Source: CAD feature listing. Evaluate the final solid. Frame: model axes, mm. Face numbers are marked on the shaded views. Coordinates: 2 decimals unless noted, no trailing zeros. Write each loop counter-clockwise with the first axis right and the second up, starting at its lowest first coordinate (ties: lowest second). Pieces come first, ordered by that corner, then holes. Notation, with made-up numbers: (66.25, 65) - (72.25, 65) arc R19 cw to (72.25, 101) - close; hole circle Ø7 at (-27, -2). An arc over 180 degrees is marked (long way). One line per question, with ' | ' between items. Start each with the question number.
Q1. Contact query for flat-ended pins moving along their axis: P1, Ø2, axis at x = -119, z = -1.5, coming from the -Y side; P2, Ø6, axis at x = 63, y = 20.5, coming from the +Z side; P3, Ø2, axis at x = 118, z = 32.5, coming from the +Y side (3 decimals). Output: stop coordinate, or through.
Q2. Cut plane D-D, the plane x = 75. Return loops of the section in (y, z) (3 decimals).
Q3. Cut plane C-C, the plane y = -7. Return loops of the section in (x, z), plus the area to 3 significant figures.
Q4. Draft query along Y for the marked faces 1 and 2. Return one class per face: +Y half, -Y half, draft (parallel to the pull), parting line (faces both ways), or undercut.
Q5. Cut plane A-A, the plane z = 45. Return loops of the section in (x, y) (3 decimals).
Q6. Line query: line 1 (X direction, y = -23, z = 24.5); line 2 (Y direction, x = -72, z = 9); line 3 (Z direction, x = -63, y = 29). Output: solid intervals per line, ascending.
Q7. Cut plane B-B, the plane x = -7. Return loops of the section in (y, z) (3 decimals).
```python
from build123d import *

# Parameters (mm, degrees)
SKETCH31_W                     = 240
SKETCH31_H                     = 80
BASE_FLANGE1_DEPTH             = 2
EDGE_FLANGE1_STRIP_W           = 9.4732
EDGE_FLANGE1_STRIP_H           = 2
EDGE_FLANGE1_STRIP_CUT_DEPTH   = 240
EDGE_FLANGE1_STRIP_2_W         = 9.4732
EDGE_FLANGE1_STRIP_2_H         = 2
EDGE_FLANGE1_STRIP_CUT_2_DEPTH = 240
EDGE_FLANGE1_DEPTH             = 240
EDGE_FLANGE1_BEND_DEPTH        = 240
EDGE_FLANGE2_STRIP_W           = 9.4732
EDGE_FLANGE2_STRIP_H           = 2
EDGE_FLANGE2_STRIP_CUT_DEPTH   = 74.5268
EDGE_FLANGE2_STRIP_2_W         = 9.4732
EDGE_FLANGE2_STRIP_2_H         = 2
EDGE_FLANGE2_STRIP_CUT_2_DEPTH = 74.5268
EDGE_FLANGE2_DEPTH             = 74.5268
EDGE_FLANGE2_BEND_DEPTH        = 74.5268
SKETCH52_W                     = 26.086706926
SKETCH52_H                     = 9.115658902
CUT_EXTRUDE2_DEPTH             = 10
SKETCH53_W                     = 26.086706926
SKETCH53_H                     = 0.049167759
CUT_EXTRUDE3_DEPTH             = 10
SKETCH61_R                     = 1.5
CUT_EXTRUDE8_DEPTH             = 167.29844137
SKETCH62_R                     = 1.5
CUT_EXTRUDE9_DEPTH             = 167.29844137
SKETCH65_W                     = 100.644593538
SKETCH65_H                     = 54.18299384
CUT_EXTRUDE11_DEPTH            = 153.543535722


# Sheet-metal steps are written as plain solids
with BuildPart() as part:
    # Base-Flange1: sheet metal written as solids
    # Sketch31 → Base-Flange1 (new body)
    with BuildSketch(Plane.XY):
        with Locations((-0.883917881, 4.881607463)):
            Rectangle(SKETCH31_W, SKETCH31_H)
    extrude(amount=-BASE_FLANGE1_DEPTH)

    # Edge-Flange1: sheet metal written as solids
    # Edge-Flange1 strip (on a plane across the edge) → Edge-Flange1 strip cut (cut)
    with BuildSketch(Plane(origin=(119.116082119, 44.881607463, 0), x_dir=(0, -1, 0), z_dir=(-1, 0, 0))):
        with Locations((-2, -1)):
            Rectangle(EDGE_FLANGE1_STRIP_W, EDGE_FLANGE1_STRIP_H)
    extrude(amount=EDGE_FLANGE1_STRIP_CUT_DEPTH, mode=Mode.SUBTRACT)

    # Edge-Flange1 strip 2 (on a plane across the edge) → Edge-Flange1 strip cut 2 (cut)
    with BuildSketch(Plane(origin=(-120.883917881, -35.118392537, 0), x_dir=(0, 1, 0), z_dir=(1, 0, 0))):
        with Locations((-2, -1)):
            Rectangle(EDGE_FLANGE1_STRIP_2_W, EDGE_FLANGE1_STRIP_2_H)
    extrude(amount=EDGE_FLANGE1_STRIP_CUT_2_DEPTH, mode=Mode.SUBTRACT)

    # Edge-Flange1 section (on a plane across the edge) → Edge-Flange1 (add)
    with BuildSketch(Plane(origin=(119.116082119, 44.881607463, 0), x_dir=(0, -1, 0), z_dir=(-1, 0, 0))):
        with BuildLine():
            Line((0, 0.7366), (0, 11))
            Line((0, 11), (2, 11))
            Line((2, 11), (2, 0.7366))
            ThreePointArc((2, 0.7366), (2.215745145, 0.215745145), (2.7366, 0))
            Line((2.7366, 0), (2.7366, -2))
            ThreePointArc((2.7366, -2), (0.801531583, -1.198468417), (0, 0.7366))
        make_face()
    extrude(amount=EDGE_FLANGE1_DEPTH)

    # Edge-Flange1 section 2 (on a plane across the edge) → Edge-Flange1 bend (add)
    with BuildSketch(Plane(origin=(-120.883917881, -35.118392537, 0), x_dir=(0, 1, 0), z_dir=(1, 0, 0))):
        with BuildLine():
            Line((0, 0.7366), (0, 11))
            Line((0, 11), (2, 11))
            Line((2, 11), (2, 0.7366))
            ThreePointArc((2, 0.7366), (2.215745145, 0.215745145), (2.7366, 0))
            Line((2.7366, 0), (2.7366, -2))
            ThreePointArc((2.7366, -2), (0.801531583, -1.198468417), (0, 0.7366))
        make_face()
    extrude(amount=EDGE_FLANGE1_BEND_DEPTH)

    # Edge-Flange2: sheet metal written as solids
    # Edge-Flange2 strip (on a plane across the edge) → Edge-Flange2 strip cut (cut)
    with BuildSketch(Plane(origin=(-120.883917881, 42.145007463, 0), x_dir=(1, 0, 0), z_dir=(0, -1, 0))):
        with Locations((-2, -1)):
            Rectangle(EDGE_FLANGE2_STRIP_W, EDGE_FLANGE2_STRIP_H)
    extrude(amount=EDGE_FLANGE2_STRIP_CUT_DEPTH, mode=Mode.SUBTRACT)

    # Edge-Flange2 strip 2 (on a plane across the edge) → Edge-Flange2 strip cut 2 (cut)
    with BuildSketch(Plane(origin=(119.116082119, -32.381792537, 0), x_dir=(-1, 0, 0), z_dir=(0, 1, 0))):
        with Locations((-2, -1)):
            Rectangle(EDGE_FLANGE2_STRIP_2_W, EDGE_FLANGE2_STRIP_2_H)
    extrude(amount=EDGE_FLANGE2_STRIP_CUT_2_DEPTH, mode=Mode.SUBTRACT)

    # Edge-Flange2 section (on a plane across the edge) → Edge-Flange2 (add)
    with BuildSketch(Plane(origin=(-120.883917881, 42.145007463, 0), x_dir=(1, 0, 0), z_dir=(0, -1, 0))):
        with BuildLine():
            Line((0, 0.7366), (0, 81.5))
            Line((0, 81.5), (2, 81.5))
            Line((2, 81.5), (2, 0.7366))
            ThreePointArc((2, 0.7366), (2.215745145, 0.215745145), (2.7366, 0))
            Line((2.7366, 0), (2.7366, -2))
            ThreePointArc((2.7366, -2), (0.801531583, -1.198468417), (0, 0.7366))
        make_face()
    extrude(amount=EDGE_FLANGE2_DEPTH)

    # Edge-Flange2 section 2 (on a plane across the edge) → Edge-Flange2 bend (add)
    with BuildSketch(Plane(origin=(119.116082119, -32.381792537, 0), x_dir=(-1, 0, 0), z_dir=(0, 1, 0))):
        with BuildLine():
            Line((0, 0.7366), (0, 81.5))
            Line((0, 81.5), (2, 81.5))
            Line((2, 81.5), (2, 0.7366))
            ThreePointArc((2, 0.7366), (2.215745145, 0.215745145), (2.7366, 0))
            Line((2.7366, 0), (2.7366, -2))
            ThreePointArc((2.7366, -2), (0.801531583, -1.198468417), (0, 0.7366))
        make_face()
    extrude(amount=EDGE_FLANGE2_BEND_DEPTH)

    # Sketch52 → Cut-Extrude2 (cut)
    with BuildSketch(Plane(origin=(0, -33.118392537, 0), x_dir=(1, 0, 0), z_dir=(0, 1, 0))):
        with Locations((-65.439575559, -6.39300279)):
            Rectangle(SKETCH52_W, SKETCH52_H)
    cut_extrude2 = extrude(amount=-CUT_EXTRUDE2_DEPTH, mode=Mode.SUBTRACT)

    # Sketch53 → Cut-Extrude3 (cut)
    with BuildSketch(Plane(origin=(0, -33.118392537, 0), x_dir=(1, 0, 0), z_dir=(0, 1, 0))):
        with Locations((-65.439575559, -10.975416121)):
            Rectangle(SKETCH53_W, SKETCH53_H)
    cut_extrude3 = extrude(amount=-CUT_EXTRUDE3_DEPTH, mode=Mode.SUBTRACT)

    # Mirror3: Cut-Extrude3 across plane
    add(cut_extrude3.mirror(Plane(origin=(0, 0, 0), x_dir=(0, 0, 1), z_dir=(1, 0, 0))), mode=Mode.SUBTRACT)

    # Mirror4: Cut-Extrude2, Cut-Extrude3 across plane
    add(cut_extrude2.mirror(Plane(origin=(0, 0, 0), x_dir=(0, 0, 1), z_dir=(1, 0, 0))), mode=Mode.SUBTRACT)
    add(cut_extrude3.mirror(Plane(origin=(0, 0, 0), x_dir=(0, 0, 1), z_dir=(1, 0, 0))), mode=Mode.SUBTRACT)

    # Sketch61 → Cut-Extrude8 (cut, through all)
    with BuildSketch(Plane(origin=(0, 44.881607463, 0), x_dir=(1, 0, 0), z_dir=(0, 1, 0))):
        with Locations(Location((111.616082119, -5.4966, 0), (0, 0, 270))):
            Circle(SKETCH61_R)
    extrude(amount=-CUT_EXTRUDE8_DEPTH, mode=Mode.SUBTRACT)

    # Sketch62 → Cut-Extrude9 (cut, through all)
    with BuildSketch(Plane(origin=(0, 44.881607463, 0), x_dir=(1, 0, 0), z_dir=(0, 1, 0))):
        with Locations(Location((-113.383917881, -5.4966, 0), (0, 0, 270))):
            Circle(SKETCH62_R)
    extrude(amount=-CUT_EXTRUDE9_DEPTH, mode=Mode.SUBTRACT)

    # Sketch65 → Cut-Extrude11 (cut, through all)
    with BuildSketch(Plane.XY):
        with Locations((-0.883917881, 4.881607463)):
            Rectangle(SKETCH65_W, SKETCH65_H)
    extrude(amount=-CUT_EXTRUDE11_DEPTH, mode=Mode.SUBTRACT)


solid = part.part
```
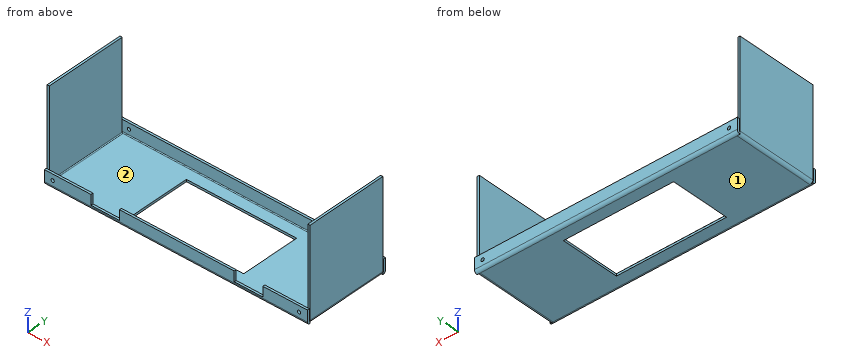
Reply:
1) P1: stops at y = -34.82 | P2: stops at z = 0 | P3: stops at y = 42.145
2) outline: (-35.118, 0.737) arc R2.737 ccw to (-32.382, -2) - (42.145, -2) arc R2.737 ccw to (44.882, 0.737) - (44.882, 11) - (42.882, 11) - (42.882, 0.737) arc R0.737 cw to (42.145, 0) - (-32.382, 0) arc R0.737 cw to (-33.118, 0.737) - (-33.118, 1.835) - (-35.118, 1.835) - close
3) outline: (-120.88, 0.74) arc R2.74 ccw to (-118.15, -2) - (-51.21, -2) - (-51.21, 0) - (-118.15, 0) arc R0.74 cw to (-118.88, 0.74) - (-118.88, 81.5) - (-120.88, 81.5) - close; (49.44, -2) - (116.38, -2) arc R2.74 ccw to (119.12, 0.74) - (119.12, 81.5) - (117.12, 81.5) - (117.12, 0.74) arc R0.74 cw to (116.38, 0) - (49.44, 0) - close | area: 602 mm^2
4) face 1: draft | face 2: undercut
5) outline: (-120.884, -32.382) - (-118.884, -32.382) - (-118.884, 42.145) - (-120.884, 42.145) - close; (117.116, -32.382) - (119.116, -32.382) - (119.116, 42.145) - (117.116, 42.145) - close
6) line 1: x = -120.88 to -118.88, 117.12 to 119.12 | line 2: y = 42.88 to 44.88 | line 3: z = -2 to 0
7) outline: (-35.118, 0.737) arc R2.737 ccw to (-32.382, -2) - (-22.21, -2) - (-22.21, 0) - (-32.382, 0) arc R0.737 cw to (-33.118, 0.737) - (-33.118, 11) - (-35.118, 11) - close; (31.973, -2) - (42.145, -2) arc R2.737 ccw to (44.882, 0.737) - (44.882, 11) - (42.882, 11) - (42.882, 0.737) arc R0.737 cw to (42.145, 0) - (31.973, 0) - close
